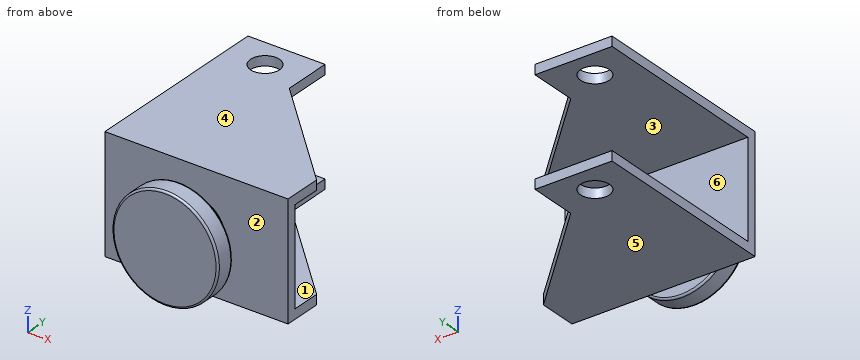
from build123d import *

# Parameters (mm, degrees)
BOSS_EXTRUDE1_DEPTH = 5
BOSS_EXTRUDE2_DEPTH = 5
SKETCH3_R           = 7.5
CUT_EXTRUDE1_DEPTH  = 149.492424049
SKETCH4_R           = 15
BOSS_EXTRUDE3_DEPTH = 12
SKETCH5_R           = 27.5
BOSS_EXTRUDE4_DEPTH = 10
FILLET1_R           = 1


with BuildPart() as part:
    # Sketch1 → Boss-Extrude1 (new body)
    with BuildSketch(Plane(origin=(0, 0, 0), x_dir=(1, 0, 0), z_dir=(0, 1, 0))):
        Polygon((0, 0), (0, 25), (95, 25), (95, -25), (0, -25), align=None)
    extrude(amount=BOSS_EXTRUDE1_DEPTH)

    # Sketch2 → Boss-Extrude2 (add)
    with BuildSketch(Plane.XY.offset(25)):
        Polygon((0, 0), (0, 100), (40, 100), (40, 75), (95, 20), (95, 0), align=None)
    boss_extrude2 = extrude(amount=BOSS_EXTRUDE2_DEPTH)

    # Sketch3 → Cut-Extrude1 (cut, through all)
    with BuildSketch(Plane.XY.offset(30)):
        with Locations((20, 85)):
            Circle(SKETCH3_R)
    cut_extrude1 = extrude(amount=-CUT_EXTRUDE1_DEPTH, mode=Mode.SUBTRACT)

    # Mirror1: Boss-Extrude2, Cut-Extrude1 across plane
    add(boss_extrude2.mirror(Plane.XY))
    add(cut_extrude1.mirror(Plane.XY), mode=Mode.SUBTRACT)

    # Sketch4 → Boss-Extrude3 (add)
    with BuildSketch(Plane(origin=(0, 0, 0), x_dir=(-1, 0, 0), z_dir=(0, -1, 0))):
        with Locations(Location((-47.5, 0, 0), (0, 0, 90))):
            Circle(SKETCH4_R)
    extrude(amount=BOSS_EXTRUDE3_DEPTH)

    # Sketch5 → Boss-Extrude4 (add)
    with BuildSketch(Plane(origin=(0, -12, 0), x_dir=(-1, 0, 0), z_dir=(0, -1, 0))):
        with Locations(Location((-47.5, 0, 0), (0, 0, 90))):
            Circle(SKETCH5_R)
    extrude(amount=BOSS_EXTRUDE4_DEPTH)

    # Fillet1
    fillet1_edges = [part.edges().sort_by_distance(p)[0] for p in [
        (47.5, -12, 27.5),
        (47.5, -22, 27.5),
    ]]
    fillet(fillet1_edges, radius=FILLET1_R)


solid = part.part
Source: CAD feature listing. Evaluate the final solid. Frame: model axes, mm. Face numbers are marked on the shaded views. A direction names the side the tool comes from. Give positions to 0.01 mm unless a question says otherwise; leave off trailing zeros. Write each loop counter-clockwise with the first axis right and the second up, starting at its lowest first coordinate (ties: lowest second). Pieces come first, ordered by that corner, then holes. Notation, with made-up numbers: M 72,-32.5 L 79,-32.5 A28 cw 79,-6.5 Z; hole C 86.25,78 d9. An arc over 180 degrees is marked long. Return JSON: item names as keys, results as strings. Group by question number.
1) Cut plane A-A, the plane y = 38.5. Output: boundary loops of the cut face in (x, z).
2) Draft query along Z for the marked faces 1, 2, 3 and 4. Return one class per face: released by +Z, released by -Z, zero draft, split by the parting line, or undercut.
3) First-contact query: pin 1 Ø17 at (x, y) = (20, 85) entering from -Z; pin 2 Ø25 at (x, z) = (49.5, 1.5) entering from +Y; pin 3 Ø1.5 at (y, z) = (82, -27) entering from +X; pin 4 Ø9 at (x, y) = (20, 85) entering from +Z. Flat tips, straight axial feed; report the tip coordinate or a pass-through.
4) Set-up query: the marked faces 5 and 6. Return all of +Z, -Z, +X, -X, +Y, -Y with unobstructed straight access to the full face (end or side cutting, diameter ignored); none if empty.
5) Cut plane B-B, the plane x = 7. Output: boundary loops of the cut face in (y, z).
6) Ray query, L1, parallel to Z at x = 24.5, y = 32; L2, parallel to Y at x = 27, z = 15.5; L3, parallel to X at y = 85, z = -28. Return the intervals inside material, ascending.
7) Cut plane D-D, the plane z = 0. Output: boundary loops of the cut face in (x, y).
8) Cut plane C-C, the plane y = 85. Output: boundary loops of the cut face in (x, z), then the cut area to 3 significant figures.
Data:
{
 "1": {"outline": "M 0,-30 L 76.5,-30 L 76.5,-25 L 0,-25 Z; M 0,25 L 76.5,25 L 76.5,30 L 0,30 Z"},
 "2": {"face 1": "undercut", "face 2": "zero draft", "face 3": "undercut", "face 4": "released by +Z"},
 "3": {"pin 1": "stops at z = -30", "pin 2": "stops at y = 5", "pin 3": "stops at x = 40", "pin 4": "passes through"},
 "4": {"face 5": "-Z, +X, -X, +Y, -Y", "face 6": "+X, -X, +Y"},
 "5": {"outline": "M 0,-30 L 100,-30 L 100,-25 L 5,-25 L 5,25 L 100,25 L 100,30 L 0,30 Z"},
 "6": {"L1": "z = -30 to -25, 25 to 30", "L2": "y = -22 to -12, 0 to 5", "L3": "x = 0 to 12.5, 27.5 to 40"},
 "7": {"outline": "M 0,0 L 32.5,0 L 32.5,-12 L 21,-12 A1 ccw 20,-13 L 20,-21 A1 ccw 21,-22 L 74,-22 A1 ccw 75,-21 L 75,-13 A1 ccw 74,-12 L 62.5,-12 L 62.5,0 L 95,0 L 95,5 L 0,5 Z"},
 "8": {"outline": "M 0,-30 L 12.5,-30 L 12.5,-25 L 0,-25 Z; M 0,25 L 12.5,25 L 12.5,30 L 0,30 Z; M 27.5,-30 L 40,-30 L 40,-25 L 27.5,-25 Z; M 27.5,25 L 40,25 L 40,30 L 27.5,30 Z", "area": "250 mm²"}
}
